Read the model definition and answer for the solid it produces. Units are mm, in the model's axes. A direction names the side the tool comes from. Give positions to 0.01 mm unless a question says otherwise; leave off trailing zeros. Write each loop counter-clockwise with the first axis right and the second up, starting at its lowest first coordinate (ties: lowest second). Pieces come first, ordered by that corner, then holes. Notation, with made-up numbers: (-33.5, 89.5) -> (-24.5, 89.5) arc R24 ccw to (-24.5, 125.5) -> close; hole circle Ø11 at (52.5, -24.5). An arc over 180 degrees is marked (long way). Write item = value, one per line.
from build123d import *

# Parameters (mm, degrees)
F5_D = 100
F7_D = 100


# Not quite as in the source:
# - a feature names something its author has since deleted; it is built from what else it names


with BuildPart() as f2:
    # F2: sweep along a path in F1
    with BuildLine(Plane.XY) as f2_path:
        Line((-107.3189526796, -226.6205847263), (-115.9728169441, -761.2517476082))
        Line((-115.9728169441, -761.2517476082), (-413.3533239365, -1301.2853860855))
    # F0 (on Front) → F2 (sweep)
    with BuildSketch(Plane.XZ):
        with BuildLine():
            Line((-836.5186393261, 158.2419019938), (-836.5186393261, 148.2419019938))
            Line((-836.5186393261, 148.2419019938), (-436.5186393261, 148.2419019938))
            Line((-436.5186393261, 148.2419019938), (-436.5186393261, 548.2419019938))
            Line((-436.5186393261, 548.2419019938), (-446.5186393261, 548.2419019938))
            ThreePointArc((-446.5186393261, 548.2419019938), (-474.8029105736, 536.5261732412), (-486.5186393261, 508.2419019938))
            Line((-486.5186393261, 508.2419019938), (-486.5186393261, 248.2419019938))
            ThreePointArc((-486.5186393261, 248.2419019938), (-501.1633002668, 212.8865629344), (-536.5186393261, 198.2419019938))
            Line((-536.5186393261, 198.2419019938), (-796.5186393261, 198.2419019938))
            ThreePointArc((-796.5186393261, 198.2419019938), (-824.8029105736, 186.5261732412), (-836.5186393261, 158.2419019938))
        make_face()
    sweep(path=f2_path.line, transition=Transition.RIGHT)

    # F3: F2 across face


with BuildPart() as f2_1:
    add(f2.part)
    add(f2.part.mirror(Plane(origin=(-700.4191524375, -892.7521403639, 263.9571660189), x_dir=(0.8836600113, -0.4681292389, 0), z_dir=(-0.4681292389, -0.8836600113, 0))))

    # F5 (through all)
    with Locations(Plane.XY.offset(198.2419019938)):
        with Locations((-667.7702069283, -149.9368995428)):
            Hole(F5_D / 2)

    # F7 (through all)
    with Locations(Plane.XY.offset(198.2419019938)):
        with Locations((-1321.2910347152, -1389.5985503476)):
            Hole(F7_D / 2)


solid = f2_1.part
(1) Given P1, Ø2, axis at x = -859.5, z = 332, coming from the +Y side; P2, Ø12, axis at y = -559.5, z = 269, coming from the +X side; P3, Ø10, axis at x = -1142, z = 417.5, coming from the -Y side, each flat-ended and moving along its own axis, determine where each tip first touches the part or whether it passes through.
Checks:
P1 = -1247.61
P2 = -445.48
P3 = -1511.49
(2) Consider L1, parallel to Z at x = -747, y = -704.5; L2, parallel to X at y = -1393.5, z = 295; L3, parallel to X at y = -1277, z = 398. Determine where each line is inside the solid, lowest interval first.
Checks:
L1 = 148.24 to 198.24
L2 = -1066.06 to -979.12
L3 = -900.31 to -813.37
(3) A tool of negligible diameter and unlimited length cuts with its end or side. For faces 1 (the flat face through (-1045.102, -1378.767, 380.062)), 2 (the flat face through (-1319.389, -1570.427, 230.657)), from which of +Z, -Z, +X, -X, +Y, -Y can it reach the whole face along a straight path? Write none if from no direction.
Checks:
face_1 = +Z, -X, +Y
face_2 = +Z, -Z, -X, -Y
(4) For a pull along X with two mould halves and no side action, classify faces 3 (the cylindrical face through (-1284.439, -1355.806, 172.892)), 4 (the flat face through (-1280.13, -1116.21, 153.31)), 5 (the flat face through (-852, -790, 198.242)) as released by +X, released by -X, zero draft, split by the parting line, or undercut.
Checks:
face_3 = undercut
face_4 = released by -X
face_5 = zero draft
(5) The part is cut by section A-A on z = 343. Determine the outline of the cut face in (x, y).
Checks:
outline = (-1318.87, -1571.19) -> (-1290.79, -1612.55) -> (-739.98, -1225.42) -> (-598.17, -946.92) -> (-447.41, -673.16) -> (-436.52, 0) -> (-486.52, 0) -> (-497.2, -659.93) -> (-642.35, -923.52) -> (-778.89, -1191.66) -> close
